Autodesk Inventor part; units mm, degrees
ref_plane "YZ Plane" through (0, 0, 0) normal (1, 0, 0) x (0, 1, 0)
ref_plane "XZ Plane" through (0, 0, 0) normal (0, 1, 0) x (-1, 0, 0)
ref_plane "XY Plane" through (0, 0, 0) normal (0, 0, 1) x (1, 0, 0)
sketch "Sketch1" plane through (0, 0, 0) normal (0, 1, 0) x (-1, 0, 0)
  line L0 (60, 45) -> (-60, 45)
  line L1 (-60, 45) -> (-60, -45)
  line L2 (-60, -45) -> (60, -45)
  line L3 (60, -45) -> (60, 45)
  point P0 (0, 0)
  point P1 (0, 0)
  dimension "d0" = 120
  dimension "d1" = 60
  dimension "d2" = 90
  dimension "d3" = 45
extrude "Plate1" add sketch "Sketch1" along normal blind 6.35
sketch "Sketch2" plane through (-53.65, 6.35, 45) normal (-1, 0, 0) x (0, 1, 0)
  line L0 (0, -90) -> (0, 0)
  line L1 (0, 0) -> (-34, 0)
  line L2 (-34, 0) -> (-34, -90)
  line L3 (-34, -90) -> (0, -90)
edge flange "Flange1" height 34 angle 90 thickness 6.35 bend radius 6.35 thickness toward (-1, 0, 0) relief tear relief width 6.35 relief depth 3.175 edges at (-60, 6.35, 0) wall of the first edge with corners at (-53.65, 6.35, -45) (-53.65, 6.35, 45) (-53.65, -27.65, 45) (-53.65, -27.65, -45)
bend "Bend1"
corner "Corner1"
sketch "Sketch4" plane through (-53.65, -21.3, -45) normal (0, -1, 0) x (-1, 0, 0)
  line L0 (0, 90) -> (0, 0)
  line L1 (0, 0) -> (30, 0)
  line L2 (30, 0) -> (30, 90)
  line L3 (30, 90) -> (0, 90)
edge flange "Flange3" height 30 angle 90 thickness 6.35 bend radius 6.35 thickness toward (0, -1, 0) relief tear relief width 6.35 relief depth 3.175 edges at (-53.65, -27.65, 0) wall of the first edge with corners at (-53.65, -21.3, 45) (-53.65, -21.3, -45) (-83.65, -21.3, -45) (-83.65, -21.3, 45)
bend "Bend3"
corner "Corner3"
sketch "Sketch5" plane through (53.65, 6.35, 45) normal (1, 0, 0) x (0, 1, 0)
  line L0 (0, -90) -> (0, 0)
  line L1 (0, 0) -> (-34, 0)
  line L2 (-34, 0) -> (-34, -90)
  line L3 (-34, -90) -> (0, -90)
edge flange "Flange4" height 34 angle 90 thickness 6.35 bend radius 6.35 thickness toward (1, 0, 0) relief tear relief width 6.35 relief depth 3.175 edges at (60, 0, 0) wall of the first edge with corners at (53.65, 6.35, -45) (53.65, 6.35, 45) (53.65, -27.65, 45) (53.65, -27.65, -45)
bend "Bend4"
corner "Corner4"
sketch "Sketch6" plane through (53.65, -21.3, 45) normal (0, -1, 0) x (-1, 0, 0)
  line L0 (0, -90) -> (0, 0)
  line L1 (0, 0) -> (-34, 0)
  line L2 (-34, 0) -> (-34, -90)
  line L3 (-34, -90) -> (0, -90)
edge flange "Flange5" height 34 angle 90 thickness 6.35 bend radius 6.35 thickness toward (0, -1, 0) relief tear relief width 6.35 relief depth 3.175 edges at (53.65, -27.65, 0) wall of the first edge with corners at (53.65, -21.3, -45) (53.65, -21.3, 45) (87.65, -21.3, 45) (87.65, -21.3, -45)
bend "Bend5"
corner "Corner5"
sketch "Sketch7" plane through (0, 6.35, 0) normal (0, 1, 0) x (1, 0, 0)
  line L0 (37.3, 18) -> (37.3, -18)
  line L1 (47.3, -45) -> (47.3, 45)
  point P0 (0, 0)
  dimension "d55" = 36
  dimension "d56" = 18
  dimension "d57" = 10
hole "Hole1" at (37.3, 6.35, -18) at (37.3, 6.35, 18) direction (0, -1, 0) diameter 10 depth 6.35
sketch "Sketch8" plane through (-83.65, -21.3, 45) normal (0, 1, 0) x (1, 0, 0)
  line L0 (17.3, 0) -> (0, 0)
  line L1 (8.65, 0) -> (8.65, 90)
  line L2 (0, 90) -> (17.3, 90)
  line L3 (0, 0) -> (0, 90)
  line L4 (0, 20) -> (17.3, 20)
  line L5 (17.3, 0) -> (17.3, 90)
  line L6 (0, 70) -> (17.3, 70)
  point P0 (83.65, 45)
  point P1 (8.65, 20)
  point P2 (8.65, 70)
  dimension "d65" = 20
  dimension "d66" = 20
hole "Hole2" at (-75, -21.3, 25) at (-75, -21.3, -25) direction (0, -1, 0) diameter 10 depth 6.35
mirror "Mirror1" about plane through (0, 0, 0) normal (1, 0, 0) of "Hole2"
equation "\"d63\" = Thickness"
equation "\"d72\" = Thickness"
equation "\"d4\" = Thickness"
equation "\"d5\" = BendReliefWidth"
equation "\"d6\" = BendReliefDepth"
equation "\"d7\" = MinimumRemnant"
equation "\"d8\" = TransitionRadius"
equation "\"d11\" = BendRadius"
equation "\"d12\" = CornerReliefSize"
equation "\"d13\" = GapSize"
equation "\"d14\" = JacobiRadiusSize"
equation "\"d25\" = BendReliefWidth"
equation "\"d26\" = BendReliefDepth"
equation "\"d27\" = MinimumRemnant"
equation "\"d28\" = TransitionRadius"
equation "\"d31\" = BendRadius"
equation "\"d32\" = CornerReliefSize"
equation "\"d33\" = GapSize"
equation "\"d34\" = JacobiRadiusSize"
equation "\"d35\" = BendReliefWidth"
equation "\"d36\" = BendReliefDepth"
equation "\"d37\" = MinimumRemnant"
equation "\"d38\" = TransitionRadius"
equation "\"d41\" = BendRadius"
equation "\"d42\" = CornerReliefSize"
equation "\"d43\" = GapSize"
equation "\"d44\" = JacobiRadiusSize"
equation "\"d45\" = BendReliefWidth"
equation "\"d46\" = BendReliefDepth"
equation "\"d47\" = MinimumRemnant"
equation "\"d48\" = TransitionRadius"
equation "\"d51\" = BendRadius"
equation "\"d52\" = CornerReliefSize"
equation "\"d53\" = GapSize"
equation "\"d54\" = JacobiRadiusSize"
equation "\"BendRadius\" = Thickness"
equation "\"BendReliefWidth\" = Thickness"
equation "\"BendReliefDepth\" = 0.5 * Thickness"
equation "\"CornerReliefSize\" = 4 * Thickness"
equation "\"MinimumRemnant\" = 2 * Thickness"
equation "\"TransitionRadius\" = BendRadius"
equation "\"JacobiRadiusSize\" = BendRadius"
equation "\"GapSize\" = Thickness"
properties part number "PlacaActuadorAvance"
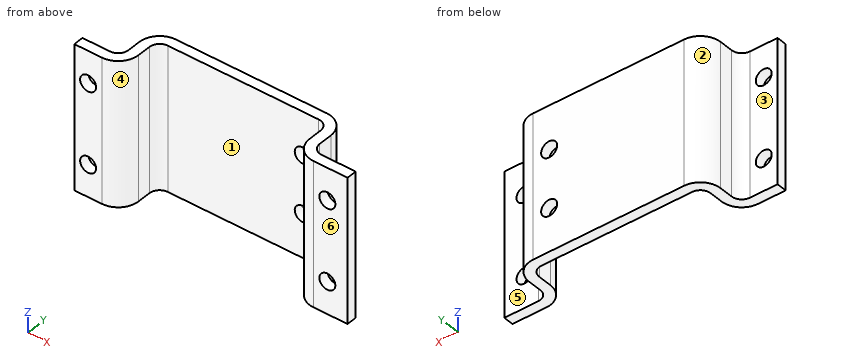
Geometry check sheet. Reference: the model listing, model coordinates, mm. Face numbers are marked on the shaded views. A direction names the side the tool comes from. Give positions to 0.01 mm unless a question says otherwise; leave off trailing zeros. Order: outer loops, then holes, each group sorted by start corner. A loop starts at its lowest first (then second) coordinate and runs counter-clockwise, first axis right, second up. Notation, with made-up numbers: (29, -26) - (61, -26) arc R31 cw to (61, 10) - close; hole circle Ø7 at (-14, -27). An arc over 180 degrees is marked (long way). Answer in a Markdown table with one row per item. Add a question column.
Q1. Cross-section at D-D, the plane z = -38. Enter the section's corners in (x, y), then the cut area to 3 significant figures.
Q2. Material ranges on probe 1 along Z at (x, y) = (37, 4); probe 2 along Z at (x, y) = (-75, -24); probe 3 along X at (y, z) = (-23, 25), recorded low to high. Write a range as from..to.
Q3. Cross-section at C-C, the plane y = -9.5. Enter the section's corners in (x, z), then the cut area to 3 significant figures.
Q4. Gauge pin test, flat ends, axial feed: pin 1 (17 mm diameter, centred on x = 78.5, z = 12, fed in from +Y); pin 2 (2.5 mm diameter, centred on y = -12.5, z = 11, fed in from -X); pin 3 (9 mm diameter, centred on x = 37.3, z = -18, fed in from +Y); pin 4 (10 mm diameter, centred on x = 5.5, z = 4, fed in from -Y). Record the tip position at first contact, or that the pin passes through.
Q5. Cross-section at B-B, the plane x = -75. Enter the section's corners in (y, z), then the cut area to 4 significant figures.
Q6. Cross-section at A-A, the plane z = 18. Enter the section's corners in (x, y), then the cut area to 3 significant figures.
Q7. Tool access check on the marked faces 4, 5 and 6. Record the directions out of +Z, -Z, +X, -X, +Y, -Y that give a thin tool (end or side, any length) a straight path to the whole face; none if there is none.
Q8. Mould release check, pull along X, two halves, no side actions. Record for the marked faces 1, 2 and 3: pulls with the +X half, pulls with the -X half, needs draft (parallel to the pull), parting line crosses it, or undercut.
Check values:
| question | item | result |
|---|---|---|
| 1 | outline | (-83.65, -27.65) - (-66.35, -27.65) arc R12.7 ccw to (-53.65, -14.95) - (-53.65, -6.35) arc R6.35 cw to (-47.3, 0) - (47.3, 0) arc R6.35 cw to (53.65, -6.35) - (53.65, -14.95) arc R12.7 ccw to (66.35, -27.65) - (87.65, -27.65) - (87.65, -21.3) - (66.35, -21.3) arc R6.35 cw to (60, -14.95) - (60, -6.35) arc R12.7 ccw to (47.3, 6.35) - (-47.3, 6.35) arc R12.7 ccw to (-60, -6.35) - (-60, -14.95) arc R6.35 cw to (-66.35, -21.3) - (-83.65, -21.3) - close |
| 1 | area | 1,340 mm^2 |
| 2 | probe 1 | z = -45..-22.99, -13.01..13.01, 22.99..45 |
| 2 | probe 2 | z = -45..-30, -20..20, 30..45 |
| 2 | probe 3 | x = -83.65..-80, -70..-56.53, 56.53..70, 80..87.65 |
| 3 | outline | (-60, -45) - (-53.65, -45) - (-53.65, 45) - (-60, 45) - close; (53.65, -45) - (60, -45) - (60, 45) - (53.65, 45) - close |
| 3 | area | 1,140 mm^2 |
| 4 | pin 1 | stops at y = -21.3 |
| 4 | pin 2 | stops at x = -60 |
| 4 | pin 3 | passes through |
| 4 | pin 4 | stops at y = 0 |
| 5 | outline | (-27.65, -45) - (-21.3, -45) - (-21.3, -30) - (-27.65, -30) - close; (-27.65, -20) - (-21.3, -20) - (-21.3, 20) - (-27.65, 20) - close; (-27.65, 30) - (-21.3, 30) - (-21.3, 45) - (-27.65, 45) - close |
| 5 | area | 444.5 mm^2 |
| 6 | outline | (-83.65, -27.65) - (-66.35, -27.65) arc R12.7 ccw to (-53.65, -14.95) - (-53.65, -6.35) arc R6.35 cw to (-47.3, 0) - (32.3, 0) - (32.3, 6.35) - (-47.3, 6.35) arc R12.7 ccw to (-60, -6.35) - (-60, -14.95) arc R6.35 cw to (-66.35, -21.3) - (-83.65, -21.3) - close; (42.3, 0) - (47.3, 0) arc R6.35 cw to (53.65, -6.35) - (53.65, -14.95) arc R12.7 ccw to (66.35, -27.65) - (87.65, -27.65) - (87.65, -21.3) - (66.35, -21.3) arc R6.35 cw to (60, -14.95) - (60, -6.35) arc R12.7 ccw to (47.3, 6.35) - (42.3, 6.35) - close |
| 6 | area | 1,270 mm^2 |
| 7 | face 4 | +Z, -Z, -Y |
| 7 | face 5 | +Z, -Z, +X, +Y |
| 7 | face 6 | +Z, -Z, +X, -X, -Y |
| 8 | face 1 | undercut |
| 8 | face 2 | pulls with the -X half |
| 8 | face 3 | needs draft |
